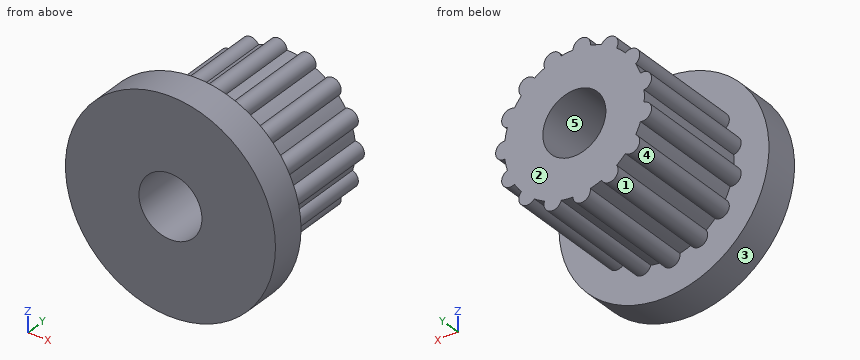
```python
from build123d import *

# Parameters (mm, degrees)
CYLINDER011034_R     = 1.8
CYLINDER011034_DEPTH = 20
CYLINDER011033_R     = 6
CYLINDER011033_DEPTH = 2
CYLINDER011035_R     = 0.5
CYLINDER011035_DEPTH = 7
ARRAY018_COUNT       = 15
CYLINDER011032_R     = 4
CYLINDER011032_DEPTH = 7


with BuildPart() as belt_attach_bolt_hole001:
    # Cylinder011034 → Cylinder011034 (new body)
    with BuildSketch(Plane.XZ):
        Circle(CYLINDER011034_R)
    extrude(amount=CYLINDER011034_DEPTH)


with BuildPart() as belt_disk001:
    # Cylinder011033 → Cylinder011033 (new body)
    with BuildSketch(Plane.XZ.offset(7)):
        Circle(CYLINDER011033_R)
    extrude(amount=CYLINDER011033_DEPTH)


with BuildPart() as belt_pin_array001:
    # Cylinder011035 → Cylinder011035 (new body)
    with BuildSketch(Plane(origin=(4, 0, 0), x_dir=(1, 0, 0), z_dir=(0, -1, 0))):
        Circle(CYLINDER011035_R)
    extrude(amount=CYLINDER011035_DEPTH)

    # Array018: belt pin array001 ×15 about axis
    array018_axis = Axis((0, 0, 0), (0, 1, 0))


with BuildPart() as belt_pin_array001_1:
    add(belt_pin_array001.part)
    for i in range(1, ARRAY018_COUNT):
        add(belt_pin_array001.part.rotate(array018_axis, i * 360 / ARRAY018_COUNT))


with BuildPart() as horizontal_belt_attach_cut:
    # Cylinder011032 → Cylinder011032 (new body)
    with BuildSketch(Plane.XZ):
        Circle(CYLINDER011032_R)
    extrude(amount=CYLINDER011032_DEPTH)

    # Fusion012: union belt disk001, belt pin array001
    add(belt_disk001.part)
    add(belt_pin_array001_1.part)

    # Cut023015009022: cut belt attach bolt hole001
    add(belt_attach_bolt_hole001.part, mode=Mode.SUBTRACT)


solid = horizontal_belt_attach_cut.part
```
The model under review builds one solid part; all positions refer to its coordinate system, in mm. Face numbers are marked on the shaded views. A direction names the side the tool comes from. Round coordinates to 2 decimals unless told otherwise and drop trailing zeros. Loops run counter-clockwise (first coordinate to the right, second up) from the corner with the lowest first, then second, coordinate; pieces in that order, holes last. Notation, with made-up numbers: M 71,-1.5 L 107,-1.5 A8 ccw 107,12.5 Z; hole C 87.5,53.25 d4. An arc over 180 degrees is marked long. Write item = value, one per line.
Item 1: Insertion check: P1, Ø2, axis at y = -2.5, z = -3.5, coming from the +X side; P2, Ø4, axis at y = -5.5, z = -4.5, coming from the -X side; P3, Ø4, axis at x = 3, y = -2.5, coming from the -Z side. Each pin has a flat end and moves straight along its axis. Give the tip position at first contact, or say it passes through.
Return value:
P1 = 3.18
P2 = -5.09
P3 = -4.3
Item 2: Take a section at D-D on x = -2. Write out the cut boundary in (y, z), then the cut area to 3 significant figures.
Return value:
outline = M -9,-5.66 L -7,-5.66 L -7,-3.96 L 0,-3.96 L 0,3.96 L -7,3.96 L -7,5.66 L -9,5.66 Z
area = 78.1 mm2
Item 3: The part is to be moulded in two halves that separate along X. For the marked faces 1, 2 and 3, say which applies: released by +X, released by -X, zero draft, split by the parting line, or undercut.
Return value:
face_1 = undercut
face_2 = zero draft
face_3 = split by the parting line
Item 4: Machinability: for the marked faces 4 and 5, which of the approach directions +Z, -Z, +X, -X, +Y, -Y give a long, thin tool a straight path to every point of the face, cutting with its end or side? Answer none if there is none.
Return value:
face_4 = +Y
face_5 = +Y, -Y
Item 5: For line 1 (Y direction, x = 0.75, z = -4.75); line 2 (Z direction, x = 0, y = -5.5); line 3 (Z direction, x = -1.25, y = -4.25), list the stretches that pass through material, from the lowest coordinate up. Write a range as [from, to].
Return value:
line_1 = [-9, -7]
line_2 = [-4.25, -1.8], [1.8, 4.25]
line_3 = [-3.8, -1.3], [1.3, 3.8]
Item 6: Take a section at B-B on z = 0. Write out the cut boundary in (x, y), then the cut area to 3 significant figures.
Return value:
outline = M -6,-9 L -1.8,-9 L -1.8,0 L -4,0 L -4,-7 L -6,-7 Z; M 1.8,-9 L 6,-9 L 6,-7 L 4.5,-7 L 4.5,0 L 1.8,0 Z
area = 51.1 mm2
Item 7: Take a section at C-C on x = 0.5. Write out the cut boundary in (y, z), then the cut area to 3 significant figures.
Return value:
outline = M -9,-5.98 L -7,-5.98 L -7,-3.97 L 0,-3.97 L 0,-1.73 L -9,-1.73 Z; M -9,1.73 L 0,1.73 L 0,3.97 L -7,3.97 L -7,5.98 L -9,5.98 Z
area = 48.4 mm2
